The model under review builds one solid part; all positions refer to its coordinate system, in mm. A direction names the side the tool comes from. Give positions to 0.01 mm unless a question says otherwise; leave off trailing zeros. Write each loop counter-clockwise with the first axis right and the second up, starting at its lowest first coordinate (ties: lowest second). Pieces come first, ordered by that corner, then holes. Notation, with made-up numbers: M 1,49 L 39,49 A10 cw 39,68 Z; hole C -34.75,-8 d8. An arc over 180 degrees is marked long. Write item = value, one per line. Start each with the question number.
```python
from build123d import *

# Parameters (mm, degrees)
ESQUISSE1_R        = 2
BOSS_EXTRU_1_DEPTH = 5
CONG_1_R           = 5


with BuildPart() as part:
    # Esquisse1 → Boss.-Extru.1 (new body)
    with BuildSketch(Plane.XY):
        Polygon((0, 0), (0, 30), (210, 30), (210, 0), (190, 0), (190, 15), (20, 15), (20, 0), align=None)
        with Locations((5, 5)):
            Circle(ESQUISSE1_R, mode=Mode.SUBTRACT)
        with Locations((205, 5)):
            Circle(ESQUISSE1_R, mode=Mode.SUBTRACT)
    extrude(amount=BOSS_EXTRU_1_DEPTH)

    # Congé1
    cong_1_edges = [part.edges().sort_by_distance(p)[0] for p in [
        (0, 0, 2.5),
        (0, 30, 2.5),
        (210, 30, 2.5),
        (210, 0, 2.5),
        (190, 0, 2.5),
        (190, 15, 2.5),
        (20, 15, 2.5),
        (20, 0, 2.5),
    ]]
    fillet(cong_1_edges, radius=CONG_1_R)


solid = part.part
```
Item 1: We need section D-D, the plane x = 187.5. Write out the cut boundary in (y, z).
Item 2: We need section C-C, the plane x = 51.5. Write out the cut boundary in (y, z).
Item 3: The part is to be moulded in two halves that separate along Y. For faces 1 (the cylindrical face through (203, 5, 2)), 2 (the cylindrical face through (3, 5, 2)), 3 (the flat face through (190, 7, 2)), 4 (the flat face through (106, 15, 2)), say which applies: released by +Y, released by -Y, zero draft, split by the parting line, or undercut.
Item 4: We need section B-B, the plane y = 12.25. Write out the cut boundary in (x, z), and give its area (3 significant figures).
Item 5: For faces 5 (the cylindrical face through (188, 14, 3)), 6 (the flat face through (10, 0, 2)), list the 3-axis set-ups (+Z, -Z, +X, -X, +Y, -Y) from which the entire face can be reached by the end or side of a thin tool; tool diameter is ignored.
Item 6: Clearance check with a flat-ended pin moving along its axis: P1, Ø3, axis at x = 5, y = 5, coming from the +Z side. State where the tip first meets the part, or that it passes through.
Item 7: We need section A-A, the plane z = 1.05. Write out the cut boundary in (x, y), and give its area (3 significant figures).
Item 8: To check wall thickness, follow probe 1 along Y at (x, z) = (5, 1.2); probe 2 along X at (y, z) = (10, 4.85); probe 3 along Y at (x, z) = (33, 0.9). State the ranges of each line that lie inside material, in increasing order. Write a range as [from, to].
Worked out:
q1.outline = M 14.33,0 L 30,0 L 30,5 L 14.33,5 Z
q2.outline = M 15,0 L 30,0 L 30,5 L 15,5 Z
q3.face_1 = undercut
q3.face_2 = undercut
q3.face_3 = zero draft
q3.face_4 = released by -Y
q4.outline = M 0,0 L 20.53,0 L 20.53,5 L 0,5 Z; M 189.47,0 L 210,0 L 210,5 L 189.47,5 Z
q4.area = 205 mm²
q5.face_5 = +Z, -Z, -Y
q5.face_6 = +Z, -Z, +X, -X, -Y
q6.P1 = through
q7.outline = M 0,5 A5 ccw 5,0 L 15,0 A5 ccw 20,5 L 20,10 A5 cw 25,15 L 185,15 A5 cw 190,10 L 190,5 A5 ccw 195,0 L 205,0 A5 ccw 210,5 L 210,25 A5 ccw 205,30 L 5,30 A5 ccw 0,25 Z; hole C 5,5 d4; hole C 205,5 d4
q7.area = 3,700 mm²
q8.probe_1 = [0, 3], [7, 30]
q8.probe_2 = [0, 20], [190, 210]
q8.probe_3 = [15, 30]
